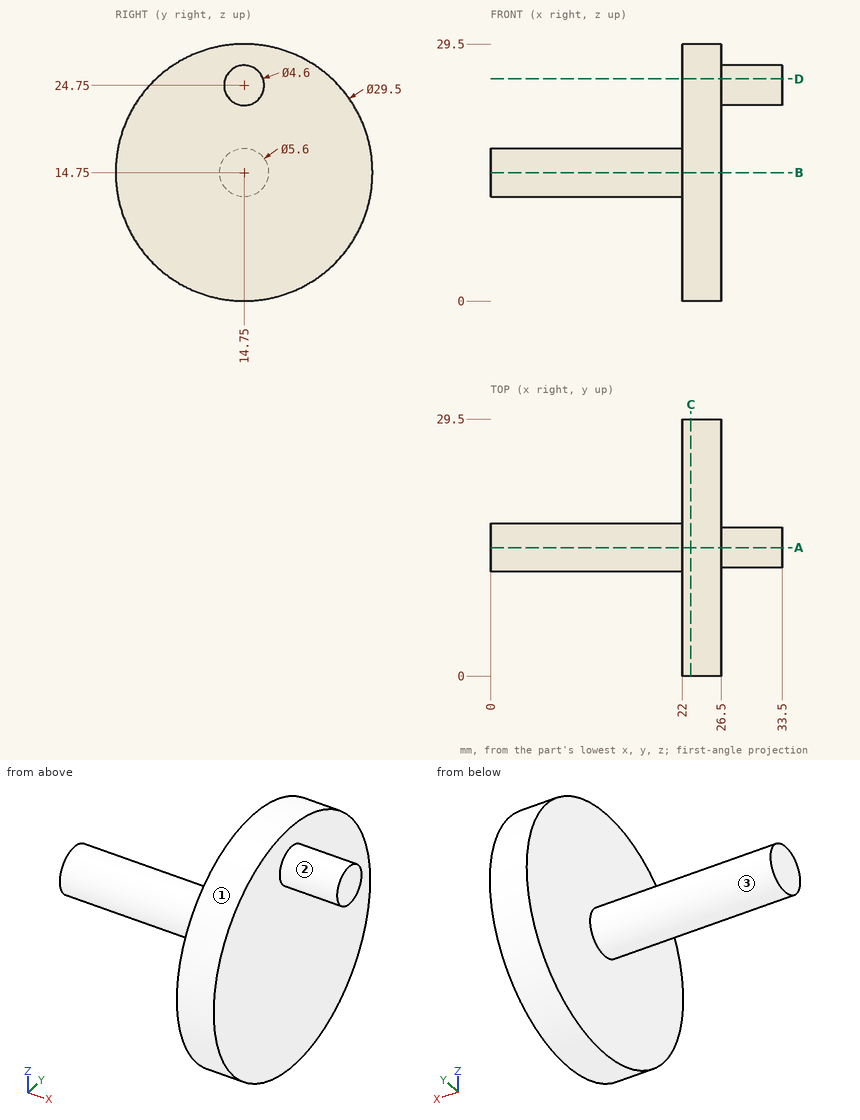
Print and shaded views of the part. All mm, measured from the part's lowest x, y and z. A direction names the side the tool comes from. Round coordinates to 2 decimals unless told otherwise and drop trailing zeros. Write each loop counter-clockwise with the first axis right and the second up, starting at its lowest first coordinate (ties: lowest second). Pieces come first, ordered by that corner, then holes. Notation, with made-up numbers: (2, 1.25) -> (38, 1.25) arc R28 ccw to (38, 24.25) -> close; hole circle Ø9 at (13.25, 51). An arc over 180 degrees is marked (long way). Return JSON: item names as keys, results as strings. Group by question number.
Q1. Which spindle directions (+Z, -Z, +X, -X, +Y, -Y) get a long thin tool onto all of the face, cutting with end or side? Do the marked faces 1, 2 and 3. Say none if no direction does.
Q2. Probe L1, parallel to X at y = 14.5, z = 8; L2, parallel to Y at x = 17.5, z = 16.25; L3, parallel to X at y = 15, z = 13.5. List the from-to ranges inside material, lowest first. Write a range as [from, to].
Q3. Saw through at D-D on z = 25.5. Write the cut outline in (x, y).
Q4. Saw through at A-A on y = 14.75. Write the cut outline in (x, z), plus the area to 3 significant figures.
Q5. Saw through at B-B on z = 14.75. Write the cut outline in (x, y).
Q6. Saw through at C-C on x = 23. Write the cut outline in (y, z).
Q7. Pin check, flat tips, straight feed: pin 1 (12 mm diameter, centred on y = 24.5, z = 11, fed in from -X); pin 2 (10 mm diameter, centred on x = 8, y = 10, fed in from +Z); pin 3 (1 mm diameter, centred on x = 25.5, y = 22, fed in from +Z). Stop position of each tip, or through.
Answer:
{
 "1": {"face 1": "+X, -X", "face 2": "+X", "face 3": "-X"},
 "2": {"L1": "[22, 26.5]", "L2": "[12.39, 17.11]", "L3": "[0, 26.5]"},
 "3": {"outline": "(22, 4.65) -> (26.5, 4.65) -> (26.5, 12.58) -> (33.5, 12.58) -> (33.5, 16.92) -> (26.5, 16.92) -> (26.5, 24.85) -> (22, 24.85) -> close"},
 "4": {"outline": "(0, 11.95) -> (22, 11.95) -> (22, 0) -> (26.5, 0) -> (26.5, 22.45) -> (33.5, 22.45) -> (33.5, 27.05) -> (26.5, 27.05) -> (26.5, 29.5) -> (22, 29.5) -> (22, 17.55) -> (0, 17.55) -> close", "area": "288 mm2"},
 "5": {"outline": "(0, 11.95) -> (22, 11.95) -> (22, 0) -> (26.5, 0) -> (26.5, 29.5) -> (22, 29.5) -> (22, 17.55) -> (0, 17.55) -> close"},
 "6": {"outline": "circle Ø29.5 at (14.75, 14.75)"},
 "7": {"pin 1": "x = 22", "pin 2": "z = 17.55", "pin 3": "z = 27.86"}
}
